Input: dimensioned drawing with shaded views. Units: mm. Origin: part minimum x, y, z. A direction names the side the tool comes from. Round coordinates to 2 decimals unless told otherwise and drop trailing zeros. Write each loop counter-clockwise with the first axis right and the second up, starting at its lowest first coordinate (ties: lowest second). Pieces come first, ordered by that corner, then holes. Notation, with made-up numbers: (-34.75, 46) - (12.25, 46) arc R28 ccw to (12.25, 69) - close; hole circle Ø1 at (87.25, 57.25). An arc over 180 degrees is marked (long way). Use one line per item in the form item = value.
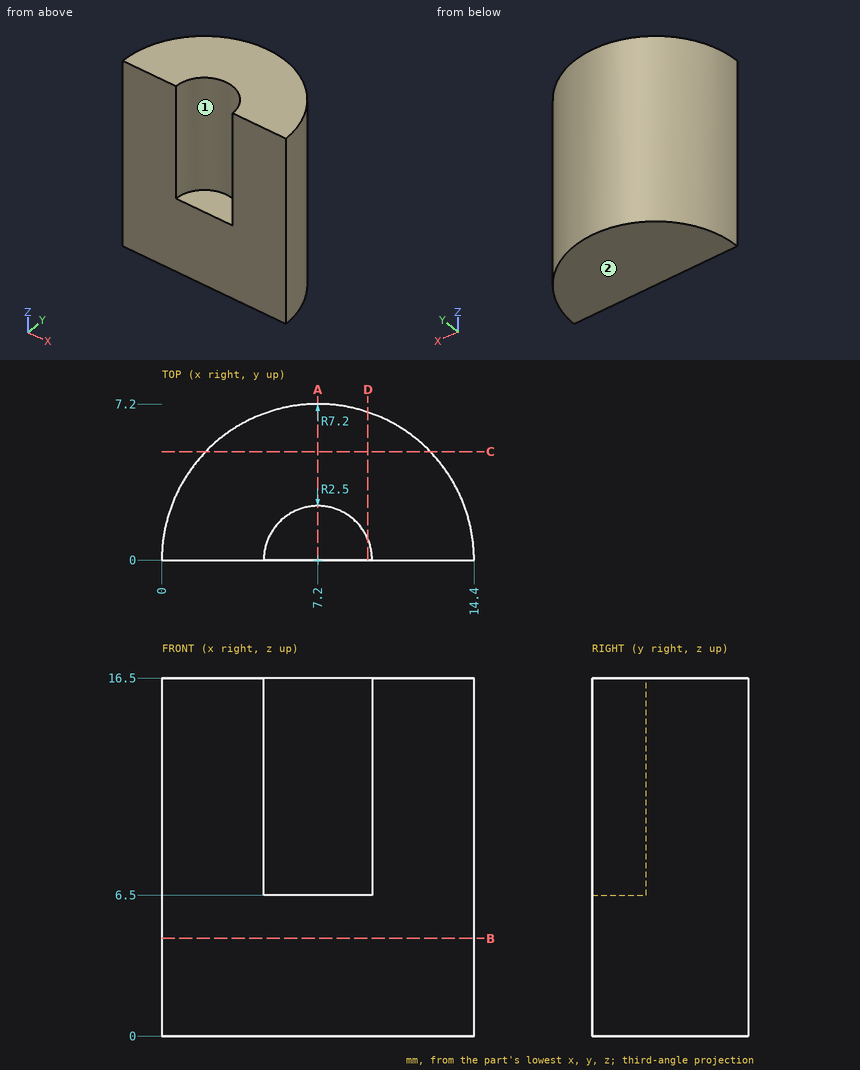
(1) Cut plane B-B on z = 4.5. Output: boundary loops of the cut face in (x, y).
Derived:
outline = (0, 0) - (14.4, 0) arc R7.2 ccw to start
(2) Cut plane C-C on y = 5. Output: boundary loops of the cut face in (x, z), then the cut area to 3 significant figures.
Derived:
outline = (2.02, 0) - (12.38, 0) - (12.38, 16.5) - (2.02, 16.5) - close
area = 171 mm^2
(3) Access query for the marked faces 1 and 2. Directions: +Z, -Z, +X, -X, +Y, -Y. A direction counts if a zero-diameter tool reaches every point of the face in a straight line with its end or side. Return the directions, or none.
Derived:
face_1 = +Z, -Y
face_2 = -Z, +X, -X, +Y, -Y
(4) Cut plane A-A on x = 7.2. Output: boundary loops of the cut face in (y, z).
Derived:
outline = (0, 0) - (7.2, 0) - (7.2, 16.5) - (2.5, 16.5) - (2.5, 6.5) - (0, 6.5) - close
(5) Material intervals for L1, parallel to Z at x = 8, y = 2.25; L2, parallel to X at y = 1, z = 14; L3, parallel to X at y = 2, z = 10.25, sorted ascending.
Derived:
L1 = 0 to 6.5
L2 = 0.07 to 4.91, 9.49 to 14.33
L3 = 0.28 to 5.7, 8.7 to 14.12
(6) First-contact query: pin 1 Ø0.8 at (x, y) = (6.5, 1.5) entering from +Z; pin 2 Ø2 at (y, z) = (1.5, 11) entering from -X; pin 3 Ø4 at (x, z) = (3, 10) entering from -Y; pin 4 Ø2 at (y, z) = (4, 2.5) entering from -X. Flat tips, straight axial feed; report the tip coordinate or a pass-through.
Derived:
pin_1 = 6.5
pin_2 = 0.02
pin_3 = 0
pin_4 = 0.65
(7) Cut plane D-D on x = 9.5. Output: boundary loops of the cut face in (y, z), then the cut area to 3 significant figures.
Derived:
outline = (0, 0) - (6.82, 0) - (6.82, 16.5) - (0.98, 16.5) - (0.98, 6.5) - (0, 6.5) - close
area = 103 mm^2
